Build history of the part. All positions in model axes, mm. Face numbers are marked on the shaded views. A direction names the side the tool comes from. Round coordinates to 2 decimals unless told otherwise and drop trailing zeros. Loops run counter-clockwise (first coordinate to the right, second up) from the corner with the lowest first, then second, coordinate; pieces in that order, holes last. Notation, with made-up numbers: (77, 50.25) - (102, 50.25) arc R10 cw to (102, 55.25) - close; hole circle Ø3 at (41.25, 78). An arc over 180 degrees is marked (long way). Use a Markdown table: item, result.
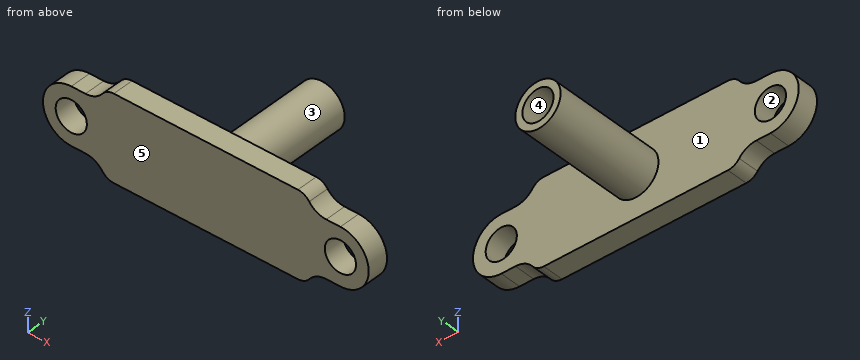
from build123d import *

# Parameters (mm, degrees)
SKETCH1_R           = 1.1
BOSS_EXTRUDE1_DEPTH = 1.5
FILLET1_R           = 1
FILLET2_R           = 1.5
SKETCH2_R           = 1.6
SKETCH2_R_2         = 1.1
BOSS_EXTRUDE2_DEPTH = 8


with BuildPart() as part:
    # Sketch1 → Boss-Extrude1 (new body)
    with BuildSketch(Plane(origin=(0, 0, 0), x_dir=(1, 0, 0), z_dir=(0, 1, 0))):
        with BuildLine():
            Line((-9.5, 2), (-7.5, 2))
            Line((-7.5, 2), (-7.5, 3))
            Line((-7.5, 3), (7.5, 3))
            Line((7.5, 3), (7.5, 2))
            Line((7.5, 2), (9.5, 2))
            ThreePointArc((9.5, 2), (11.5, 0), (9.5, -2))
            Line((9.5, -2), (7.5, -2))
            Line((7.5, -2), (7.5, -3))
            Line((7.5, -3), (-7.5, -3))
            Line((-7.5, -3), (-7.5, -2))
            Line((-7.5, -2), (-9.5, -2))
            ThreePointArc((-9.5, -2), (-11.5, 0), (-9.5, 2))
        make_face()
        with Locations(Location((-9.5, 0, 0), (0, 0, 270))):
            Circle(SKETCH1_R, mode=Mode.SUBTRACT)
        with Locations(Location((9.5, 0, 0), (0, 0, 90))):
            Circle(SKETCH1_R, mode=Mode.SUBTRACT)
    extrude(amount=BOSS_EXTRUDE1_DEPTH)

    # Fillet1
    fillet1_edges = [part.edges().sort_by_distance(p)[0] for p in [
        (7.5, 0.75, 3),
        (7.5, 0.75, -3),
        (-7.5, 0.75, -3),
        (-7.5, 0.75, 3),
    ]]
    fillet(fillet1_edges, radius=FILLET1_R - 0.0001)  # a hair under: the kernel refuses the full size

    # Fillet2
    fillet2_edges = [part.edges().sort_by_distance(p)[0] for p in [
        (7.5, 0.75, -2),
        (7.5, 0.75, 2),
        (-7.5, 0.75, 2),
        (-7.5, 0.75, -2),
    ]]
    fillet(fillet2_edges, radius=FILLET2_R)

    # Sketch2 → Boss-Extrude2 (add)
    with BuildSketch(Plane(origin=(0, 1.5, 0), x_dir=(1, 0, 0), z_dir=(0, 1, 0))):
        with Locations(Location((0, 0, 0), (0, 0, 270))):
            Circle(SKETCH2_R)
        with Locations(Location((0, 0, 0), (0, 0, 270))):
            Circle(SKETCH2_R_2, mode=Mode.SUBTRACT)
    extrude(amount=BOSS_EXTRUDE2_DEPTH)


solid = part.part
Q1. Drop flat-ended pins along their axis: pin 1 (1.1 mm diameter, centred on x = -9, y = 0.5, fed in from -Z); pin 2 (1.3 mm diameter, centred on x = 9.5, z = 0, fed in from -Y); pin 3 (1 mm diameter, centred on x = -3.5, z = -2, fed in from +Y); pin 4 (1.5 mm diameter, centred on x = 1.5, y = 3, fed in from +Z). Give the stop position or say it passes through.
Results found:
| item | result |
|---|---|
| pin 1 | stops at z = -2 |
| pin 2 | passes through |
| pin 3 | stops at y = 1.5 |
| pin 4 | stops at z = 1.41 |
Q2. Cut at C-C, the plane y = 6.5. List the corners of the cut face in (x, z).
Results found:
| item | result |
|---|---|
| outline | circle Ø3.2 at (0, 0); hole circle Ø2.2 at (0, 0) |
Q3. Cut at A-A, the plane z = 0. List the corners of the cut face in (x, y).
Results found:
| item | result |
|---|---|
| outline | (-11.5, 0) - (-10.6, 0) - (-10.6, 1.5) - (-11.5, 1.5) - close; (-8.4, 0) - (8.4, 0) - (8.4, 1.5) - (1.6, 1.5) - (1.6, 9.5) - (1.1, 9.5) - (1.1, 1.5) - (-1.1, 1.5) - (-1.1, 9.5) - (-1.6, 9.5) - (-1.6, 1.5) - (-8.4, 1.5) - close; (10.6, 0) - (11.5, 0) - (11.5, 1.5) - (10.6, 1.5) - close |
Q4. Cut at B-B, the plane x = 0. List the corners of the cut face in (y, z).
Results found:
| item | result |
|---|---|
| outline | (0, -3) - (1.5, -3) - (1.5, -1.6) - (9.5, -1.6) - (9.5, -1.1) - (1.5, -1.1) - (1.5, 1.1) - (9.5, 1.1) - (9.5, 1.6) - (1.5, 1.6) - (1.5, 3) - (0, 3) - close |
Q5. Probe line 1 (X direction, y = 1.05, z = 0); line 2 (Z direction, x = 9.5, y = 0.7); line 3 (X direction, y = 3.5, z = 0). List the from-to ranges inside material, lowest first.
Results found:
| item | result |
|---|---|
| line 1 | x = -11.5 to -10.6, -8.4 to 8.4, 10.6 to 11.5 |
| line 2 | z = -2 to -1.1, 1.1 to 2 |
| line 3 | x = -1.6 to -1.1, 1.1 to 1.6 |
Q6. Pull direction Z, two halves, no side cores. Call the marked faces 1, 2 and 3: pulls with the +Z half, pulls with the -Z half, needs draft (parallel to the pull), parting line crosses it, or undercut.
Results found:
| item | result |
|---|---|
| face 1 | needs draft |
| face 2 | undercut |
| face 3 | parting line crosses it |
Q7. Which spindle directions (+Z, -Z, +X, -X, +Y, -Y) get a long thin tool onto all of the face, cutting with end or side? Do the marked faces 4 and 5. Say none if no direction does.
Results found:
| item | result |
|---|---|
| face 4 | +Y |
| face 5 | +Z, -Z, +X, -X, -Y |
Q8. Cut at D-D, the plane x = -8.75. List the corners of the cut face in (y, z), plus the area to 3 significant figures.
Results found:
| item | result |
|---|---|
| outline | (0, -2) - (1.5, -2) - (1.5, -0.8) - (0, -0.8) - close; (0, 0.8) - (1.5, 0.8) - (1.5, 2) - (0, 2) - close |
| area | 3.59 mm2 |
